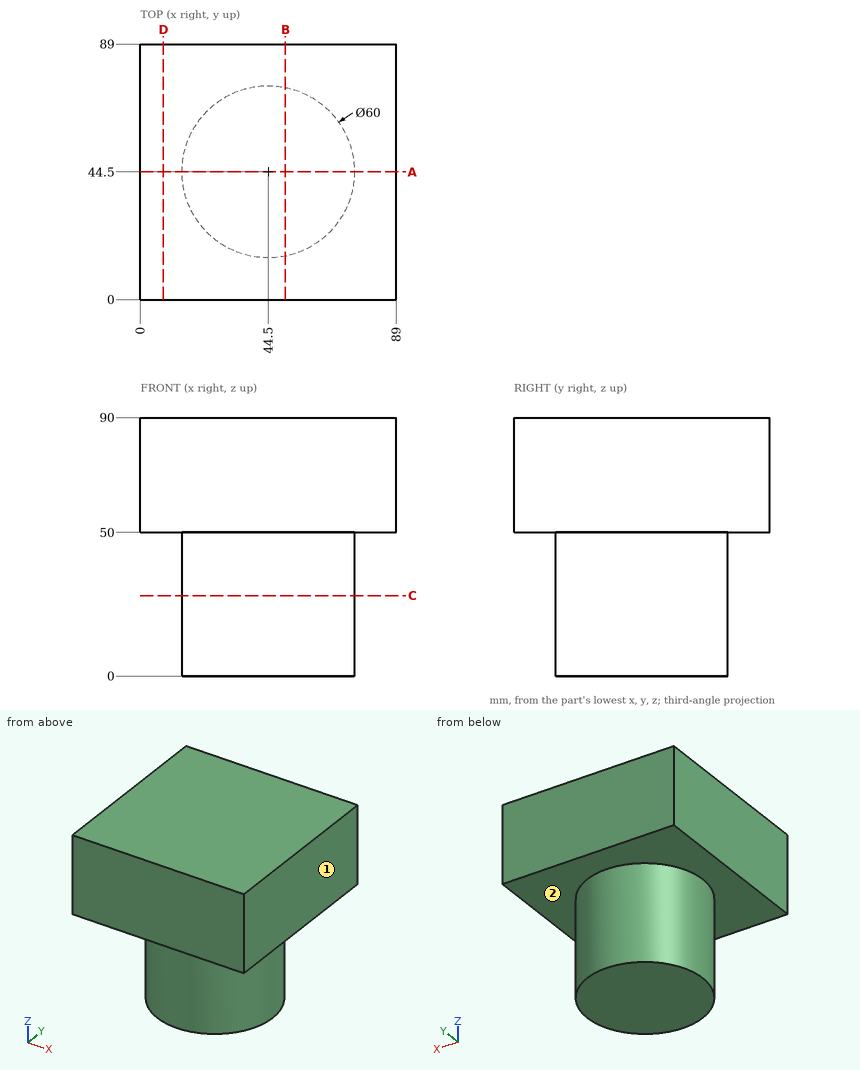
The figure shows three views and two pictorial views of one solid part (mm, origin at its lowest corner). Answer the questions. A direction names the side the tool comes from. Coordinates: 2 decimals unless noted, no trailing zeros. Loops run counter-clockwise (first coordinate to the right, second up) from the corner with the lowest first, then second, coordinate; pieces in that order, holes last. Notation, with made-up numbers: (63, 1.5) -> (69, 1.5) arc R13 cw to (69, 20.5) -> close; hole circle Ø2 at (19.5, 86.25). An arc over 180 degrees is marked (long way). Return JSON: item names as keys, results as strings. Group by question number.
(1) Find the intervals of material crossed by probe 1 along Z at (x, y) = (36.5, 8.5); probe 2 along X at (y, z) = (57.5, 39.5); probe 3 along Y at (x, z) = (24.5, 40.5), in increasing order. Write a range as from..to.
(2) A cutting plane is placed at D-D on x = 8. Write down the section's boundary in (y, z).
(3) A cutting plane is placed at B-B on x = 50.5. Write down the section's boundary in (y, z), and give its area (3 significant figures).
(4) Given pin 1 Ø1.5 at (y, z) = (69, 46) entering from -X; pin 2 Ø6 at (y, z) = (73, 27.5) entering from -X; pin 3 Ø8 at (y, z) = (37, 10.5) entering from +X, each flat-ended and moving along its own axis, determine where each tip first touches the part or whether it passes through.
(5) A cutting plane is placed at C-C on z = 28. Write down the section's boundary in (x, y), and give its area (3 significant figures).
(6) A cutting plane is placed at A-A on y = 44.5. Write down the section's boundary in (x, z).
(7) Which of the six approach directions +Z, -Z, +X, -X, +Y, -Y give full straight-line access (tool end or side, diameter ignored) to the marked faces 1 and 2?
The answers:
{
 "1": {"probe 1": "z = 50..90", "probe 2": "x = 17.46..71.54", "probe 3": "y = 22.14..66.86"},
 "2": {"outline": "(0, 50) -> (89, 50) -> (89, 90) -> (0, 90) -> close"},
 "3": {"outline": "(0, 50) -> (15.11, 50) -> (15.11, 0) -> (73.89, 0) -> (73.89, 50) -> (89, 50) -> (89, 90) -> (0, 90) -> close", "area": "6,500 mm^2"},
 "4": {"pin 1": "stops at x = 26.17", "pin 2": "stops at x = 28.7", "pin 3": "stops at x = 74.3"},
 "5": {"outline": "circle Ø60 at (44.5, 44.5)", "area": "2,830 mm^2"},
 "6": {"outline": "(0, 50) -> (14.5, 50) -> (14.5, 0) -> (74.5, 0) -> (74.5, 50) -> (89, 50) -> (89, 90) -> (0, 90) -> close"},
 "7": {"face 1": "+Z, -Z, +X, +Y, -Y", "face 2": "-Z"}
}
